The listing builds one solid part. Answer for the finished solid, in the listing's coordinates (mm). A direction names the side the tool comes from. Round coordinates to 2 decimals unless told otherwise and drop trailing zeros. Loops run counter-clockwise (first coordinate to the right, second up) from the corner with the lowest first, then second, coordinate; pieces in that order, holes last. Notation, with made-up numbers: (84.25, 10.5) -> (88.25, 10.5) arc R24 ccw to (88.25, 23.5) -> close; hole circle Ø6 at (-13.5, 83.5). An arc over 180 degrees is marked (long way). One line per question, with ' | ' between items.
Autodesk Fusion 360 part; units mm, degrees
sketch "Sketch1" plane through (0, 0, 0) normal (0, 0, 1) x (1, 0, 0)
  line L0 (46.75, 27.5) -> (-46.75, 27.5)
  line L1 (-75, 14.5) -> (-75, -14.5)
  line L2 (-46.75, -27.5) -> (46.75, -27.5)
  line L3 (75, -14.5) -> (75, 14.5)
  line L4 (75, 27.5) -> (-75, -27.5) construction
  line L5 (-75, 27.5) -> (75, -27.5) construction
  line L6 (-46.75, 27.5) -> (-46.75, 14.5)
  line L7 (-46.75, 14.5) -> (-75, 14.5)
  line L8 (46.75, 27.5) -> (46.75, 14.5)
  line L9 (46.75, 14.5) -> (75, 14.5)
  line L10 (-46.75, -27.5) -> (-46.75, -14.5)
  line L11 (-46.75, -14.5) -> (-75, -14.5)
  line L12 (46.75, -27.5) -> (46.75, -14.5)
  line L13 (46.75, -14.5) -> (75, -14.5)
  circle A0 centre (-41.75, 22.75) radius 1.75
  circle A1 centre (41.75, 22.75) radius 1.75
  circle A2 centre (-41.75, -22.75) radius 1.75
  circle A3 centre (41.75, -22.75) radius 1.75
  circle A4 centre (-61.75, 9) radius 1.25
  circle A5 centre (-61.75, -9) radius 1.25
  circle A6 centre (61.75, 9) radius 1.25
  circle A7 centre (61.75, -9) radius 1.25
  circle A8 centre (-18, 20) radius 1.75
  circle A9 centre (18, 20) radius 1.75
  circle A10 centre (-18, -20) radius 1.75
  circle A11 centre (18, -20) radius 1.75
  line L14 (2.5, 21) -> (-2.5, 21)
  line L15 (-2.5, 21) -> (-2.5, 19)
  line L16 (-2.5, 19) -> (2.5, 19)
  line L17 (2.5, 19) -> (2.5, 21)
  line L18 (2.5, 21) -> (-2.5, 19) construction
  line L19 (-2.5, 21) -> (2.5, 19) construction
  line L20 (2.5, -19) -> (-2.5, -19)
  line L21 (-2.5, -19) -> (-2.5, -21)
  line L22 (-2.5, -21) -> (2.5, -21)
  line L23 (2.5, -21) -> (2.5, -19)
  line L24 (2.5, -19) -> (-2.5, -21) construction
  line L25 (-2.5, -19) -> (2.5, -21) construction
  point P0 (0, 20)
  point P1 (0, -20)
  dimension "d1" = 150
  dimension "d2" = 55
  dimension "d3" = 28.25
  dimension "d4" = 13
  dimension "d5" = 28.25
  dimension "d6" = 13
  dimension "d7" = 28.25
  dimension "d8" = 13
  dimension "d9" = 28.25
  dimension "d10" = 13
  dimension "d11" = 3.5
  dimension "d12" = 3.5
  dimension "d13" = 3.5
  dimension "d14" = 3.5
  dimension "d15" = 2.5
  dimension "d16" = 2.5
  dimension "d17" = 2.5
  dimension "d18" = 2.5
  dimension "d19" = 4.75
  dimension "d20" = 5
  dimension "d21" = 5
  dimension "d22" = 4.75
  dimension "d23" = 5
  dimension "d24" = 4.75
  dimension "d25" = 4.75
  dimension "d26" = 5
  dimension "d29" = 13.25
  dimension "d30" = 13.25
  dimension "d33" = 13.25
  dimension "d34" = 13.25
  dimension "d35" = 18
  dimension "d36" = 18
  dimension "d37" = 3.5
  dimension "d38" = 3.5
  dimension "d39" = 3.5
  dimension "d40" = 3.5
  dimension "d41" = 7.5
  dimension "d42" = 7.5
  dimension "d45" = 7.5
  dimension "d46" = 7.5
  dimension "d49" = 5
  dimension "d50" = 2
  dimension "d51" = 5
  dimension "d52" = 2
extrude "Extrude1" add sketch "Sketch1" along normal blind 3
fillet "Fillet1" radius 1 4 edges at (46.75, -27.5, 1.5) (46.75, -14.5, 1.5) (75, -14.5, 1.5) (75, 14.5, 1.5)
fillet "Fillet2" radius 1 8 edges at (46.75, 14.5, 1.5) (46.75, 27.5, 1.5) (-46.75, 27.5, 1.5) (-75, 14.5, 1.5) (-46.75, 14.5, 1.5) (-75, -14.5, 1.5) (-46.75, -27.5, 1.5) (-46.75, -14.5, 1.5)
Q1. For faces 4 (the face through (61, 14.5, 1)), 5 (the face through (-1, 0, 3)), 6 (the face through (-46.75, -21, 1)), 7 (the face through (0, -21, 1)), determine the directions among +Z, -Z, +X, -X, +Y, -Y from which every point of the face is accessible in a straight line to the end or side of a thin tool.
Numbers:
face 4: +Z, -Z, +X, +Y | face 5: +Z, +X, -X, +Y, -Y | face 6: +Z, -Z, -X, -Y | face 7: +Z, -Z
Q2. Find the intervals of material crossed by line 1 (Y direction, x = 41.75, z = 1.8); line 2 (Y direction, x = -18, z = 1.8); line 3 (X direction, y = 8, z = 0.7), in increasing order. Write a range as from..to.
Numbers:
line 1: -27.5..-24.5, -21..21, 24.5..27.5 | line 2: -27.5..-21.75, -18.25..18.25, 21.75..27.5 | line 3: -75..-62.5, -61..61, 62.5..75
Q3. A cutting plane is placed at B-B on z = 2.5. Give the number of separate pieces and of enclosed holes in the cut face, plus the area to 3 significant figures.
Numbers:
separate pieces: 1 | enclosed holes: 14 | area: 6,660 mm^2
Q4. For a pull along Y with two mould halves and no side action, classify faces 1 (the face through (1, 27.5, 1)), 2 (the face through (42.691, -24.226, 1.479)), 3 (the face through (75, 0, 1)) as pulls with the +Y half, pulls with the -Y half, needs draft (parallel to the pull), parting line crosses it, or undercut.
Numbers:
face 1: pulls with the +Y half | face 2: undercut | face 3: needs draft
Q5. Given pin 1 Ø1.5 at (y, z) = (22.5, 1) entering from +X; pin 2 Ø1.5 at (x, z) = (-54.5, 0.5) entering from +Y; pin 3 Ø3 at (x, y) = (41.75, 22.75) entering from -Z; pin 4 Ø1.5 at (x, z) = (-47, 2) entering from +Y, each flat-ended and moving along its own axis, determine where each tip first touches the part or whether it passes through.
Numbers:
pin 1: x = 46.75 | pin 2: y = 14.5 | pin 3: through | pin 4: y = 27.37
Q6. A cutting plane is placed at A-A on x = 41.75. Give the vertices of the cut face in (y, z), plus the area to 3 significant figures.
Numbers:
outline: (-27.5, 0) -> (-24.5, 0) -> (-24.5, 3) -> (-27.5, 3) -> close; (-21, 0) -> (21, 0) -> (21, 3) -> (-21, 3) -> close; (24.5, 0) -> (27.5, 0) -> (27.5, 3) -> (24.5, 3) -> close | area: 144 mm^2
